Can you work these out from the model? Positions are in its coordinate system, mm. A direction names the side the tool comes from. Round coordinates to 2 decimals unless told otherwise and drop trailing zeros. Write each loop counter-clockwise with the first axis right and the second up, starting at its lowest first coordinate (ties: lowest second). Pieces come first, ordered by that corner, then holes. Notation, with made-up numbers: (66, 21) - (82, 21) arc R11 ccw to (82, 35) - close; hole circle Ø8 at (-8, 3). An arc over 180 degrees is marked (long way). One line per item, written item: value. Start each with the question number.
(1) Thinking about a two-plate mould opening in Y: for faces 3 (the face through (326, 5.082, -7)), 4 (the face through (326, -42.594, -6)), 5 (the face through (660.4, -20, 4)), which applies, +Y half, -Y half, draft (parallel to the pull), parting line (faces both ways), or undercut?
(2) I want a section at A-A on x = 581. List the corners of the cut face in (y, z) for me.
(3) On a 3-axis mill with a long thin cutter (end or side, diameter ignored), from which of +Z, -Z, +X, -X, +Y, -Y can I reach the whole of each face in a straight line? I mean faces 1 (the face through (326, -20, 3.103)), 2 (the face through (0, -20, 4)). Say none if no direction works.
(4) I want a section at C-C on z = -5.75. List the corners of the cut face in (x, y) for me.
(5) If I drill on L1, parallel to Y at x = 155, z = -0.75; L2, parallel to Z at x = 350.5, y = -24.5, over which ranges is the centre line in solid material (lowest first)? Write a range as from..to.
(6) I want a section at B-B on y = -22.5. List the corners of the cut face in (x, z) for me.
Autodesk Inventor part; units mm, degrees
ref_plane "YZ Plane" through (0, 0, 0) normal (1, 0, 0) x (0, 1, 0)
ref_plane "XZ Plane" through (0, 0, 0) normal (0, 1, 0) x (-1, 0, 0)
ref_plane "XY Plane" through (0, 0, 0) normal (0, 0, 1) x (1, 0, 0)
sketch "Sketch1" plane through (0, 0, 0) normal (1, 0, 0) x (0, 1, 0)
  line L0 (5.0816, 6.2276) -> (-45.7184, 6.2276)
  line L1 (-45.7184, 6.2276) -> (-45.7184, -19.1724)
  line L2 (-45.7184, -19.1724) -> (5.0816, -19.1724)
  line L3 (5.0816, -19.1724) -> (5.0816, 6.2276)
  line L4 (1.9574, 3.1034) -> (-42.5942, 3.1034)
  line L5 (-42.5942, 3.1034) -> (-42.5942, -16.0482)
  line L6 (-42.5942, -16.0482) -> (1.9574, -16.0482)
  line L7 (1.9574, -16.0482) -> (1.9574, 3.1034)
  point P0 (0, 0)
  dimension "d0" = 50.8
  dimension "d1" = 25.4
  dimension "d2" = 3.1242
extrude "Extrusion1" add sketch "Sketch1" along normal blind 660.4
properties part number "26in box beam"
Established:
1. face 3: +Y half
1. face 4: undercut
1. face 5: draft
2. outline: (-45.72, -19.17) - (5.08, -19.17) - (5.08, 6.23) - (-45.72, 6.23) - close; hole (-42.59, -16.05) - (1.96, -16.05) - (1.96, 3.1) - (-42.59, 3.1) - close
3. face 1: +X, -X
3. face 2: +Z, -Z, -X, +Y, -Y
4. outline: (0, -45.72) - (660.4, -45.72) - (660.4, -42.59) - (0, -42.59) - close; (0, 1.96) - (660.4, 1.96) - (660.4, 5.08) - (0, 5.08) - close
5. L1: -45.72..-42.59, 1.96..5.08
5. L2: -19.17..-16.05, 3.1..6.23
6. outline: (0, -19.17) - (660.4, -19.17) - (660.4, -16.05) - (0, -16.05) - close; (0, 3.1) - (660.4, 3.1) - (660.4, 6.23) - (0, 6.23) - close
